The drawing under review shows one solid part. Ordinate dimensions are in mm from its lowest x, y, z. A direction names the side the tool comes from. Round coordinates to 2 decimals unless told otherwise and drop trailing zeros. Write each loop counter-clockwise with the first axis right and the second up, starting at its lowest first coordinate (ties: lowest second). Pieces come first, ordered by that corner, then holes. Notation, with made-up numbers: (-5.75, 57.5) -> (49.25, 57.5) arc R14 cw to (49.25, 69.5) -> close; hole circle Ø5 at (81.25, -30). An arc over 180 degrees is marked (long way). Use CSV: the item, a comma, the result in double quotes. Start each with the question number.
1) Mouldability with a two-part tool opening along X and no side actions: class the marked faces 3 and 4 as released by +X, released by -X, zero draft, split by the parting line, or undercut.
2) Wall thickness on probe 1 along Z at (x, y) = (421, 33); probe 2 along Z at (x, y) = (66.5, 388.5); probe 3 along Z at (x, y) = (80.5, 220): over which ranges is each line inside the solid? List them lowest first. Write a range as [from, to].
3) For pin 1 Ø3 at (x, y) = (835.5, 550) entering from +Z; pin 2 Ø5 at (x, y) = (521.5, 218.5) entering from -Z; pin 3 Ø23 at (x, z) = (46.5, 689.5) entering from -Y, all flat-tipped, find the tip position at first contact; note any pin that passes through.
4) Take a section at C-C, the plane z = 252.5. Give the boundary of the cut face in (x, y).
5) Machinability: for the marked faces 1 and 2, which of the approach directions +Z, -Z, +X, -X, +Y, -Y give a long, thin tool a straight path to every point of the face, cutting with its end or side? Answer none if there is none.
6) Take a section at A-A, the plane x = 163. Give the boundary of the cut face in (y, z).
7) Take a section at B-B, the plane y = 260. Give the boundary of the cut face in (x, z), then the cut area to 3 significant figures.
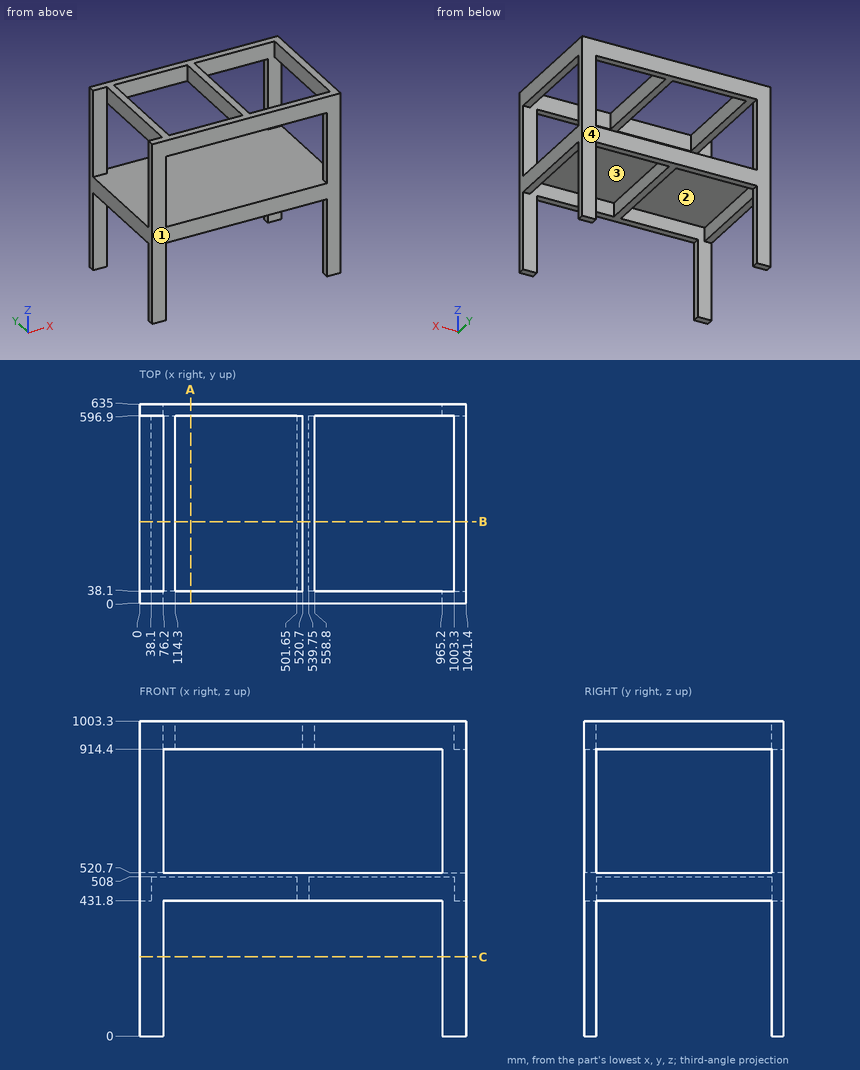
Values found:
1,face 3,"undercut"
1,face 4,"zero draft"
2,probe 1,"[431.8, 520.7], [914.4, 1003.3]"
2,probe 2,"[508, 520.7]"
2,probe 3,"[508, 520.7], [914.4, 1003.3]"
3,pin 1,"z = 520.7"
3,pin 2,"z = 431.8"
3,pin 3,"y = 0"
4,outline,"(0, 0) -> (76.2, 0) -> (76.2, 38.1) -> (0, 38.1) -> close; (0, 596.9) -> (76.2, 596.9) -> (76.2, 635) -> (0, 635) -> close; (965.2, 0) -> (1041.4, 0) -> (1041.4, 38.1) -> (965.2, 38.1) -> close; (965.2, 596.9) -> (1041.4, 596.9) -> (1041.4, 635) -> (965.2, 635) -> close"
5,face 1,"+Z, -Z, +X, -X, -Y"
5,face 2,"-Z"
6,outline,"(0, 431.8) -> (38.1, 431.8) -> (38.1, 508) -> (596.9, 508) -> (596.9, 431.8) -> (635, 431.8) -> (635, 520.7) -> (0, 520.7) -> close; (0, 914.4) -> (38.1, 914.4) -> (38.1, 1003.3) -> (0, 1003.3) -> close; (596.9, 914.4) -> (635, 914.4) -> (635, 1003.3) -> (596.9, 1003.3) -> close"
7,outline,"(0, 431.8) -> (38.1, 431.8) -> (38.1, 508) -> (501.65, 508) -> (501.65, 431.8) -> (539.75, 431.8) -> (539.75, 508) -> (1003.3, 508) -> (1003.3, 431.8) -> (1041.4, 431.8) -> (1041.4, 520.7) -> (0, 520.7) -> close; (76.2, 914.4) -> (114.3, 914.4) -> (114.3, 1003.3) -> (76.2, 1003.3) -> close; (520.7, 914.4) -> (558.8, 914.4) -> (558.8, 1003.3) -> (520.7, 1003.3) -> close; (1003.3, 914.4) -> (1041.4, 914.4) -> (1041.4, 1003.3) -> (1003.3, 1003.3) -> close"
7,area,"32,100 mm²"
